Work out the finished part from the listing and answer in its coordinate system (mm). A direction names the side the tool comes from. Give positions to 0.01 mm unless a question says otherwise; leave off trailing zeros. Loops run counter-clockwise (first coordinate to the right, second up) from the corner with the lowest first, then second, coordinate; pieces in that order, holes last. Notation, with made-up numbers: (89, 60.25) - (118, 60.25) arc R17 cw to (118, 71.25) - close; hole circle Ø6 at (-25.75, 10.5). An arc over 180 degrees is marked (long way). Use CSV: the item, a comma, the result in double quotes.
from build123d import *

# Parameters (mm, degrees)
REVOLVE1_ANGLE = 20


with BuildPart() as part:
    # Sketch1 → Revolve1 (revolve)
    with BuildSketch(Plane.XY):
        Polygon((19.05, 0), (6.35, 50.8), (0, 50.8), (0, 0), (12.7, 0), (12.7, -14.2875), (0, -14.2875), (0, -20.6375), (19.05, -20.6375), align=None)
    revolve(axis=Axis((-104.775, 37.30546868, 0), (0, -1, 0)), revolution_arc=REVOLVE1_ANGLE)


solid = part.part
Item 1: A cutting plane is placed at A-A on x = -1.25. Determine the outline of the cut face in (y, z), and give its area (3 significant figures).
Determined:
outline,"(-20.64, 16.14) - (-14.29, 16.14) - (-14.29, 37.68) - (-20.64, 37.68) - close; (0, 16.14) - (50.8, 16.14) - (50.8, 37.68) - (0, 37.68) - close"
area,"1,230 mm²"
Item 2: Given P1, Ø8, axis at x = -3.5, y = 7.5, coming from the +Z side; P2, Ø8, axis at y = -0.5, z = 17.5, coming from the +X side; P3, Ø12, axis at y = 23.5, z = 32, coming from the +X side, each flat-ended and moving along its own axis, determine where each tip first touches the part or whether it passes through.
Determined:
P1,"stops at z = 38.32"
P2,"stops at x = 18.31"
P3,"stops at x = 10.95"
Item 3: A cutting plane is placed at C-C on y = 11. Determine the outline of the cut face in (x, z) (3 decimals).
Determined:
outline,"(-6.319, 35.835) arc R104.775 cw to (0, 0) - (16.3, 0) arc R121.075 ccw to (8.998, 41.41) - close"
Item 4: A cutting plane is placed at B-B on y = -7. Determine the outline of the cut face in (x, z) (3 decimals).
Determined:
outline,"(5.615, 40.179) arc R117.475 cw to (12.7, 0) - (19.05, 0) arc R123.825 ccw to (11.582, 42.351) - close"
Item 5: For faces 1 (the flat face through (5, -14.288, 20)), 2 (the flat face through (7, 16, 0)), determine the directions among +Z, -Z, +X, -X, +Y, -Y from which every point of the face is accessible in a straight line to the end or side of a thin tool.
Determined:
face 1,"-Z, -X"
face 2,"-Z, +X, -X, +Y, -Y"
Item 6: The mould has two halves that part along Y. Classify faces 3 (the flat face through (3, 0, 20)), 4 (the flat face through (7, -20.637, 21)), 5 (the flat face through (0.518, 15.581, 38.323)): pulls with the +Y half, pulls with the -Y half, needs draft (parallel to the pull), parting line crosses it, or undercut.
Determined:
face 3,"undercut"
face 4,"pulls with the -Y half"
face 5,"needs draft"
Item 7: Find the intervals of material crossed by line 1 (Y direction, x = 4, z = 11); line 2 (X direction, y = -7.5, z = 30); line 3 (X direction, y = 18, z = 7), in increasing order.
Determined:
line 1,"y = -20.64 to -14.29, 0 to 50.8"
line 2,"x = 8.8 to 15.36"
line 3,"x = -0.23 to 14.34"
